from build123d import *

# Parameters (mm, degrees)
F1_DEPTH = 12.7
F2_W     = 8.837395
F2_H     = 77.327222
F3_DEPTH = 40
F4_R     = 13.98028
F5_DEPTH = 91.531181


with BuildPart() as f1:
    # F0 (on Top) → F1 (new body)
    with BuildSketch(Plane.XY):
        Polygon((-45.765091, 38.663611), (-45.765091, 0), (-45.765091, -38.663611), (0, -38.663611), (45.765091, -38.663611), (45.765091, 0), (45.765091, 38.663611), (0, 38.663611), align=None)
    extrude(amount=F1_DEPTH)

    # F2 (on face) → F3 (join)
    with BuildSketch(Plane.XY.offset(12.7)):
        with Locations((41.346393, 0)):
            Rectangle(F2_W, F2_H)
        with Locations((-41.346393, 0)):
            Rectangle(F2_W, F2_H)
    extrude(amount=F3_DEPTH)

    # F4 (on face) → F5 (cut, through all)
    with BuildSketch(Plane.YZ.offset(45.765091)):
        Polygon((-38.663611, 52.7), (-38.663611, 25.395), (-16.096687, 52.7), align=None)
        with Locations((17.04355, 32.666806)):
            Circle(F4_R)
    extrude(amount=-F5_DEPTH, mode=Mode.SUBTRACT)


solid = f1.part
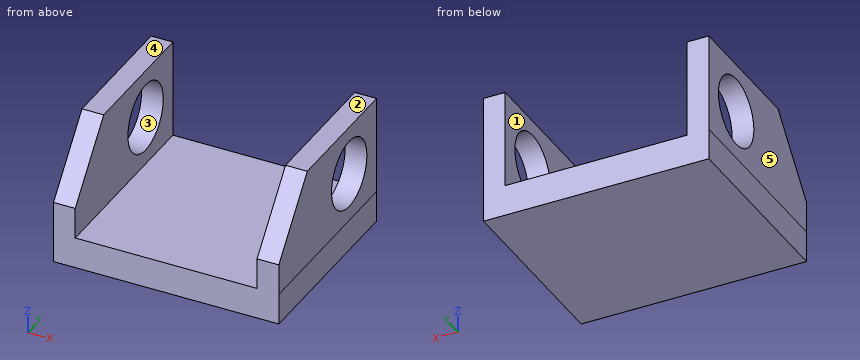
Design review of the part built by this model. Coordinates are the model's own, in mm. Face numbers are marked on the shaded views. A direction names the side the tool comes from. Round coordinates to 2 decimals unless told otherwise and drop trailing zeros. Write each loop counter-clockwise with the first axis right and the second up, starting at its lowest first coordinate (ties: lowest second). Pieces come first, ordered by that corner, then holes. Notation, with made-up numbers: (61, 44) -> (76, 44) arc R36 cw to (76, 80) -> close; hole circle Ø7 at (76.5, 10.25). An arc over 180 degrees is marked (long way). One line per item, written item: value. Start each with the question number.
Q1. Add section A-A (z = 15). Give the boundary of the cut face in (x, y).
Q2. The part is to be moulded in two halves that separate along Z. For the marked faces 3, 4 and 5, say which applies: pulls with the +Z half, pulls with the -Z half, needs draft (parallel to the pull), parting line crosses it, or undercut.
Q3. Add section B-B (y = 5.5). Give the boundary of the cut face in (x, z), then the cut area to 3 significant figures.
Q4. Add section D-D (y = -18.5). Give the boundary of the cut face in (x, z).
Q5. Add section C-C (z = 42). Give the boundary of the cut face in (x, y), then the cut area to 3 significant figures.
Q6. To check wall thickness, follow probe 1 along X at (y, z) = (-18.5, 22.5); probe 2 along Z at (x, y) = (11.5, -1); probe 3 along Z at (x, y) = (38, 22.5). State the ranges of each line that lie inside material, in increasing order.
Q7. Insertion check: P1, Ø22, axis at x = 14.5, y = -15, coming from the +Z side. The pin has a flat end and moves straight along its axis. Give the tip position at first contact, or say it passes through.
Q8. Tool access review of the marked faces 1 and 2: name each direction out of +Z, -Z, +X, -X, +Y, -Y from which nothing blocks a thin tool from reaching the whole face with its end or side.
Response:
1. outline: (-45.77, -38.66) -> (-36.93, -38.66) -> (-36.93, 38.66) -> (-45.77, 38.66) -> close; (36.93, -38.66) -> (45.77, -38.66) -> (45.77, 38.66) -> (36.93, 38.66) -> close
2. face 3: undercut
2. face 4: pulls with the +Z half
2. face 5: needs draft
3. outline: (-45.77, 0) -> (45.77, 0) -> (45.77, 24.78) -> (36.93, 24.78) -> (36.93, 12.7) -> (-36.93, 12.7) -> (-36.93, 24.78) -> (-45.77, 24.78) -> close; (-45.77, 40.55) -> (-36.93, 40.55) -> (-36.93, 52.7) -> (-45.77, 52.7) -> close; (36.93, 40.55) -> (45.77, 40.55) -> (45.77, 52.7) -> (36.93, 52.7) -> close
3. area: 1,590 mm^2
4. outline: (-45.77, 0) -> (45.77, 0) -> (45.77, 49.79) -> (36.93, 49.79) -> (36.93, 12.7) -> (-36.93, 12.7) -> (-36.93, 49.79) -> (-45.77, 49.79) -> close
5. outline: (-45.77, -24.94) -> (-36.93, -24.94) -> (-36.93, 6.63) -> (-45.77, 6.63) -> close; (-45.77, 27.45) -> (-36.93, 27.45) -> (-36.93, 38.66) -> (-45.77, 38.66) -> close; (36.93, -24.94) -> (45.77, -24.94) -> (45.77, 6.63) -> (36.93, 6.63) -> close; (36.93, 27.45) -> (45.77, 27.45) -> (45.77, 38.66) -> (36.93, 38.66) -> close
5. area: 756 mm^2
6. probe 1: x = -45.77 to -36.93, 36.93 to 45.77
6. probe 2: z = 0 to 12.7
6. probe 3: z = 0 to 19.8, 45.54 to 52.7
7. P1: stops at z = 12.7
8. face 1: +Z, +Y, -Y
8. face 2: +Z, +X, -X, +Y, -Y
